from build123d import *

# Parameters (mm, degrees)
F0_R     = 42.5
F0_R_2   = 35.5
F1_DEPTH = 8
F2_DEPTH = 50
F3_DEPTH = 4


with BuildPart() as f1:
    # F0 (on Top) → F1 (new body)
    with BuildSketch(Plane.XY):
        with Locations((26.75, -15.44412)):
            Circle(F0_R)
        with Locations((26.75, -15.44412)):
            Circle(F0_R_2, mode=Mode.SUBTRACT)
        with Locations((26.75, -15.44412)):
            Circle(F0_R_2)
        with BuildLine():
            ThreePointArc((1.125, -1.948557), (-1.948557, 1.125), (2.25, 0))
            Line((2.25, 0), (26.75, 0))
            Line((26.75, 0), (51.25, 0))
            ThreePointArc((51.25, 0), (53.5, 2.25), (55.75, 0))
            ThreePointArc((55.75, 0), (54.625, -1.948557), (52.375, -1.948557))
            Line((52.375, -1.948557), (40.125, -23.16618))
            Line((40.125, -23.16618), (27.875, -44.383802))
            ThreePointArc((27.875, -44.383802), (28.698557, -45.207359), (29, -46.332359))
            ThreePointArc((29, -46.332359), (25.625, -48.280916), (25.625, -44.383802))
            Line((25.625, -44.383802), (13.375, -23.16618))
            Line((13.375, -23.16618), (1.125, -1.948557))
        make_face(mode=Mode.SUBTRACT)
        with BuildLine():
            Line((26.75, -15.44412), (13.375, -23.16618))
            Line((13.375, -23.16618), (25.625, -44.383802))
            ThreePointArc((25.625, -44.383802), (26.167657, -44.159026), (26.75, -44.082359))
            Line((26.75, -44.082359), (26.75, -15.44412))
        make_face()
        with BuildLine():
            ThreePointArc((1.948557, -1.125), (1.59099, -1.59099), (1.125, -1.948557))
            Line((1.125, -1.948557), (13.375, -23.16618))
            Line((13.375, -23.16618), (26.75, -15.44412))
            Line((26.75, -15.44412), (1.948557, -1.125))
        make_face()
        with BuildLine():
            Line((51.551443, -1.125), (26.75, -15.44412))
            Line((26.75, -15.44412), (40.125, -23.16618))
            Line((40.125, -23.16618), (52.375, -1.948557))
            ThreePointArc((52.375, -1.948557), (51.90901, -1.59099), (51.551443, -1.125))
        make_face()
        with BuildLine():
            Line((51.25, 0), (26.75, 0))
            Line((26.75, 0), (26.75, -15.44412))
            Line((26.75, -15.44412), (51.551443, -1.125))
            ThreePointArc((51.551443, -1.125), (51.326667, -0.582343), (51.25, 0))
        make_face()
        with BuildLine():
            Line((40.125, -23.16618), (26.75, -15.44412))
            Line((26.75, -15.44412), (26.75, -44.082359))
            ThreePointArc((26.75, -44.082359), (27.332343, -44.159026), (27.875, -44.383802))
            Line((27.875, -44.383802), (40.125, -23.16618))
        make_face()
        with BuildLine():
            Line((26.75, 0), (2.25, 0))
            ThreePointArc((2.25, 0), (2.173333, -0.582343), (1.948557, -1.125))
            Line((1.948557, -1.125), (26.75, -15.44412))
            Line((26.75, -15.44412), (26.75, 0))
        make_face()
    extrude(amount=F1_DEPTH)

    # F0 (on Top) → F2 (join)
    with BuildSketch(Plane.XY):
        with Locations((26.75, -15.44412)):
            Circle(F0_R)
        with Locations((26.75, -15.44412)):
            Circle(F0_R_2, mode=Mode.SUBTRACT)
    extrude(amount=F2_DEPTH)

    # F0 (on Top) → F3 (cut)
    with BuildSketch(Plane.XY):
        with Locations((26.75, -15.44412)):
            Circle(F0_R_2)
        with BuildLine():
            ThreePointArc((1.125, -1.948557), (-1.948557, 1.125), (2.25, 0))
            Line((2.25, 0), (26.75, 0))
            Line((26.75, 0), (51.25, 0))
            ThreePointArc((51.25, 0), (53.5, 2.25), (55.75, 0))
            ThreePointArc((55.75, 0), (54.625, -1.948557), (52.375, -1.948557))
            Line((52.375, -1.948557), (40.125, -23.16618))
            Line((40.125, -23.16618), (27.875, -44.383802))
            ThreePointArc((27.875, -44.383802), (28.698557, -45.207359), (29, -46.332359))
            ThreePointArc((29, -46.332359), (25.625, -48.280916), (25.625, -44.383802))
            Line((25.625, -44.383802), (13.375, -23.16618))
            Line((13.375, -23.16618), (1.125, -1.948557))
        make_face(mode=Mode.SUBTRACT)
        with BuildLine():
            Line((26.75, 0), (2.25, 0))
            ThreePointArc((2.25, 0), (2.173333, -0.582343), (1.948557, -1.125))
            Line((1.948557, -1.125), (26.75, -15.44412))
            Line((26.75, -15.44412), (26.75, 0))
        make_face()
        with BuildLine():
            Line((51.25, 0), (26.75, 0))
            Line((26.75, 0), (26.75, -15.44412))
            Line((26.75, -15.44412), (51.551443, -1.125))
            ThreePointArc((51.551443, -1.125), (51.326667, -0.582343), (51.25, 0))
        make_face()
        with BuildLine():
            Line((26.75, -15.44412), (13.375, -23.16618))
            Line((13.375, -23.16618), (25.625, -44.383802))
            ThreePointArc((25.625, -44.383802), (26.167657, -44.159026), (26.75, -44.082359))
            Line((26.75, -44.082359), (26.75, -15.44412))
        make_face()
        with BuildLine():
            ThreePointArc((1.948557, -1.125), (1.59099, -1.59099), (1.125, -1.948557))
            Line((1.125, -1.948557), (13.375, -23.16618))
            Line((13.375, -23.16618), (26.75, -15.44412))
            Line((26.75, -15.44412), (1.948557, -1.125))
        make_face()
        with BuildLine():
            Line((51.551443, -1.125), (26.75, -15.44412))
            Line((26.75, -15.44412), (40.125, -23.16618))
            Line((40.125, -23.16618), (52.375, -1.948557))
            ThreePointArc((52.375, -1.948557), (51.90901, -1.59099), (51.551443, -1.125))
        make_face()
        with BuildLine():
            Line((40.125, -23.16618), (26.75, -15.44412))
            Line((26.75, -15.44412), (26.75, -44.082359))
            ThreePointArc((26.75, -44.082359), (27.332343, -44.159026), (27.875, -44.383802))
            Line((27.875, -44.383802), (40.125, -23.16618))
        make_face()
    extrude(amount=F3_DEPTH, mode=Mode.SUBTRACT)


solid = f1.part
Here's how the part is built. I have some questions about the finished solid (model axes, mm). A direction names the side the tool comes from. Coordinates: 2 decimals unless noted, no trailing zeros. Loops run counter-clockwise (first coordinate to the right, second up) from the corner with the lowest first, then second, coordinate; pieces in that order, holes last.
1. Imagine slicing it at A-A, the plane x = 0. Please give me the cut outline in (y, z).
2. For P1, Ø12, axis at x = 24, y = -45.5, coming from the +Z side; P2, Ø12, axis at y = -4, z = 28, coming from the -X side; P3, Ø3, axis at x = 27, z = 34, coming from the +Y side; P4, Ø1.5, axis at y = -49, z = 24.5, coming from the -X side, each with a flat end and sliding along its axis, tell me the tip position at first contact or that it passes through.
3. If we mould it in two halves opening along Y, with no side actions, what happens to faces 1 (the flat face through (17, -50, 50)), 2 (the cylindrical face through (-1.42, -37.05, 28.71)), 3 (the cylindrical face through (-1.42, -37.05, 1.97)), 4 (the cylindrical face through (67.29, -2.68, 24.65))? For each: pulls with the +Y half, pulls with the -Y half, needs draft (parallel to the pull), parting line crosses it, or undercut.
4. Imagine slicing it at D-D, the plane y = 11.5. Please give me the cut outline in (x, z).
5. Imagine slicing it at C-C, the plane x = 30.5. Please give me the cut outline in (y, z).
6. I need wall thicknesses on L1, parallel to Y at x = 26.75, z = 27.5; L2, parallel to X at y = -16, z = 34; L3, parallel to Y at x = 26.75, z = 7. Which ranges of each line are inside material? Lowest first, please.
7. Imagine slicing it at B-B, the plane y = -47.5. Please give me the cut outline in (x, z).
8. For faces 5 (the flat face through (17, -50, 0)), 6 (the flat face through (26, -15, 8)), 7 (the flat face through (26, -15, 4)), which set-ups out of +Z, -Z, +X, -X, +Y, -Y let a thin tool reach every point of the face, with its end or its side?
Taken from the geometry:
1. outline: (-48.47, 0) - (-38.78, 0) - (-38.78, 4) - (-2.25, 4) - (-2.25, 8) - (-38.78, 8) - (-38.78, 50) - (-48.47, 50) - close; (2.25, 4) - (7.89, 4) - (7.89, 0) - (17.58, 0) - (17.58, 50) - (7.89, 50) - (7.89, 8) - (2.25, 8) - close
2. P1: stops at z = 50
2. P2: stops at x = -15.4
2. P3: stops at y = 27.06
2. P4: stops at x = -0.27
3. face 1: needs draft
3. face 2: undercut
3. face 3: undercut
3. face 4: parting line crosses it
4. outline: (-6.12, 0) - (3.64, 0) - (3.64, 4) - (49.86, 4) - (49.86, 0) - (59.62, 0) - (59.62, 50) - (49.86, 50) - (49.86, 8) - (3.64, 8) - (3.64, 50) - (-6.12, 50) - close
5. outline: (-57.78, 0) - (-50.75, 0) - (-50.75, 4) - (19.86, 4) - (19.86, 0) - (26.89, 0) - (26.89, 50) - (19.86, 50) - (19.86, 8) - (-50.75, 8) - (-50.75, 50) - (-57.78, 50) - close
6. L1: y = -57.94 to -50.94, 20.06 to 27.06
6. L2: x = -15.75 to -8.75, 62.25 to 69.25
6. L3: y = -57.94 to -48.58, -44.08 to 27.06
7. outline: (-1.15, 0) - (11.5, 0) - (11.5, 4) - (24.83, 4) - (24.83, 8) - (11.5, 8) - (11.5, 50) - (-1.15, 50) - close; (28.67, 4) - (42, 4) - (42, 0) - (54.65, 0) - (54.65, 50) - (42, 50) - (42, 8) - (28.67, 8) - close
8. face 5: -Z, +X, -X, +Y, -Y
8. face 6: +Z
8. face 7: -Z
